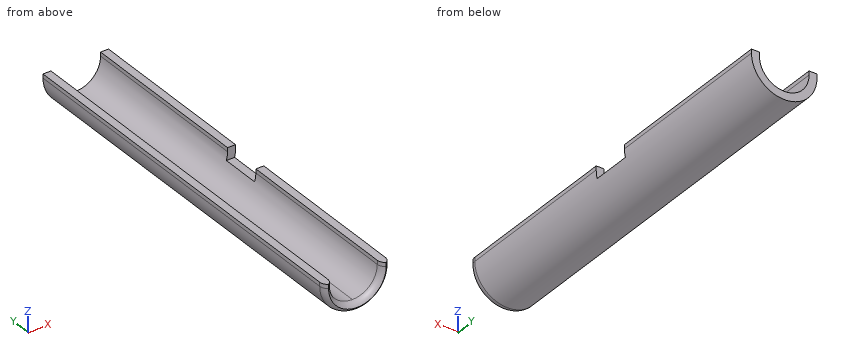
```python
from build123d import *

# Parameters (mm, degrees)
F1_DEPTH    = 127
F2_W        = 12.7
F2_H        = 2.54
F2_H_2      = 1.27
F3_DEPTH    = 9.525
F4_T1_DEPTH = 7.62
F4_T4_ANGLE = 180
F4_T6_ANGLE = 180


# Not quite as in the source:
# - a fillet or chamfer that OpenCascade refuses, or shapes differently, is made with other operations: its cross-section is extruded or revolved along the edge and cut away or added


with BuildPart() as f1:
    # F0 (on Front) → F1 (new body)
    with BuildSketch(Plane.XZ):
        with BuildLine():
            ThreePointArc((0, -7.9375), (-5.6126600757, -5.6126600757), (-7.9375, 0))
            Line((-7.9375, 0), (-7.9375, 1.27))
            Line((-7.9375, 1.27), (-10.4775, 1.27))
            Line((-10.4775, 1.27), (-10.4775, 0))
            ThreePointArc((-10.4775, 0), (0, -10.4775), (10.4775, 0))
            Line((10.4775, 0), (10.4775, 1.27))
            Line((10.4775, 1.27), (7.9375, 1.27))
            Line((7.9375, 1.27), (7.9375, 0))
            ThreePointArc((7.9375, 0), (5.6126600757, -5.6126600757), (0, -7.9375))
        make_face()
    extrude(amount=F1_DEPTH)

    # F2 (on face) → F3 (cut)
    with BuildSketch(Plane.YZ.offset(10.4775)):
        with Locations((-63.5, -1.27)):
            Rectangle(F2_W, F2_H)
        with Locations((-63.5, 0.635)):
            Rectangle(F2_W, F2_H_2)
    extrude(amount=-F3_DEPTH, mode=Mode.SUBTRACT)

    # F4: fillet of radius 2.54 on 2 edges, made by hand

    # F4_s2 → F4_t1 (cut)
    with BuildSketch(Plane.XY):
        with BuildLine():
            ThreePointArc((-10.4775, -124.46), (-9.7335512242, -126.2560512242), (-7.9375, -127))
            Line((-7.9375, -127), (-10.4775, -127))
            Line((-10.4775, -127), (-10.4775, -124.46))
        make_face()
        with BuildLine():
            ThreePointArc((10.4775, -124.46), (9.7335512242, -126.2560512242), (7.9375, -127))
            Line((7.9375, -127), (10.4775, -127))
            Line((10.4775, -127), (10.4775, -124.46))
        make_face()
        with BuildLine():
            ThreePointArc((-7.9375, -124.46), (-8.6814487758, -126.2560512242), (-10.4775, -127))
            Line((-10.4775, -127), (-7.9375, -127))
            Line((-7.9375, -127), (-7.9375, -124.46))
        make_face()
        with BuildLine():
            ThreePointArc((10.4775, -127), (8.6814487758, -126.2560512242), (7.9375, -124.46))
            Line((7.9375, -124.46), (7.9375, -127))
            Line((7.9375, -127), (10.4775, -127))
        make_face()
    extrude(amount=F4_T1_DEPTH, mode=Mode.SUBTRACT)

    # F4_s3 → F4_t4 (revolve, cut)
    with BuildSketch(Plane.XY):
        with BuildLine():
            ThreePointArc((-7.9375, -124.46), (-8.6814487758, -126.2560512242), (-10.4775, -127))
            Line((-10.4775, -127), (-7.9375, -127))
            Line((-7.9375, -127), (-7.9375, -124.46))
        make_face()
    revolve(axis=Axis((0, -127, 0), (0, -1, 0)), revolution_arc=F4_T4_ANGLE, mode=Mode.SUBTRACT)

    # F4_s5 → F4_t6 (revolve, cut)
    with BuildSketch(Plane.XY):
        with BuildLine():
            ThreePointArc((-10.4775, -124.46), (-9.7335512242, -126.2560512242), (-7.9375, -127))
            Line((-7.9375, -127), (-10.4775, -127))
            Line((-10.4775, -127), (-10.4775, -124.46))
        make_face()
    revolve(axis=Axis((0, -127, 0), (0, -1, 0)), revolution_arc=F4_T6_ANGLE, mode=Mode.SUBTRACT)


solid = f1.part
```
Source: CAD feature listing. Evaluate the final solid. Frame: model axes, mm. Give positions to 0.01 mm unless a question says otherwise; leave off trailing zeros. Loops run counter-clockwise (first coordinate to the right, second up) from the corner with the lowest first, then second, coordinate; pieces in that order, holes last. Notation, with made-up numbers: (-25.75, 24.5) -> (16.25, 24.5) arc R14 cw to (16.25, 35.5) -> close; hole circle Ø8 at (-37.5, 12). An arc over 180 degrees is marked (long way). Put each result on its own line as item: value. Start each with the question number.
1) Cut plane A-A (y = -51.5). Return loops of the section in (x, z) (1 decimal).
2) Contact query for flat-ended pins moving along their axis: P1, Ø3.5, axis at x = 9, z = 0, coming from the +Y side; P2, Ø4, axis at x = 3.5, y = -37.5, coming from the +Z side; P3, Ø1, axis at y = -36.5, z = -8, coming from the -X side; P4, Ø3, axis at y = -65, z = -5, coming from the -X side. Output: stop coordinate, or through.
3) Material intervals for probe 1 along X at (y, z) = (-43.5, 0.25); probe 2 along X at (y, z) = (-84.5, -0.75); probe 3 along X at (y, z) = (-62.5, 0.75), sorted ascending.
Results are:
1. outline: (-10.5, 0) arc R10.5 ccw to (10.5, 0) -> (10.5, 1.3) -> (7.9, 1.3) -> (7.9, 0) arc R7.9 cw to (-7.9, 0) -> (-7.9, 1.3) -> (-10.5, 1.3) -> close
2. P1: stops at y = 0
2. P2: stops at z = -5.72
2. P3: stops at x = -7.32
2. P4: stops at x = -9.88
3. probe 1: x = -10.48 to -7.94, 7.94 to 10.48
3. probe 2: x = -10.45 to -7.9, 7.9 to 10.45
3. probe 3: x = -10.48 to -7.94
